from build123d import *

# Parameters (mm, degrees)
F1_DEPTH = 63.5
F0_W     = 25.4
F0_H     = 19.05
F2_DEPTH = 25.4
F3_DEPTH = 7.9375
F5_R     = 5.08
F6_DEPTH = 46.736


with BuildPart() as f1:
    # F0 (on Front) → F1 (new body, symmetric)
    with BuildSketch(Plane.XZ):
        Polygon((22.225, 9.525), (-41.275, 9.525), (-41.275, -9.525), (41.275, -9.525), (41.275, 9.525), align=None)
    extrude(amount=F1_DEPTH, both=True)

    # F0 (on Front) → F2 (join, symmetric)
    with BuildSketch(Plane.XZ):
        with BuildLine():
            Line((22.225, 27.0002), (22.225, 9.525))
            Line((22.225, 9.525), (41.275, 9.525))
            Line((41.275, 9.525), (41.275, 27.0002))
            ThreePointArc((41.275, 27.0002), (45.9246798487, 38.2255201513), (57.15, 42.8752))
            Line((57.15, 42.8752), (60.325, 42.8752))
            Line((60.325, 42.8752), (60.325, 61.9252))
            Line((60.325, 61.9252), (57.15, 61.9252))
            add(Edge.make_bspline(
                [(53.8854342407, 61.7722898912), (54.9842067368, 61.8365871986), (56.0728453275, 61.8876096574), (57.15, 61.9252)],
                knots=[108.5245810491, 108.5245810491, 108.5245810491, 108.5245810491, 111.5045361635, 111.5045361635, 111.5045361635, 111.5045361635], degree=3))
            ThreePointArc((53.8854342407, 61.7722898912), (31.3258777096, 50.5133948686), (22.225, 27.0002))
        make_face()
        with Locations((73.025, 52.4002)):
            Rectangle(F0_W, F0_H)
    extrude(amount=F2_DEPTH, both=True)

    # F0 (on Front) → F3 (join, symmetric)
    with BuildSketch(Plane.XZ):
        with BuildLine():
            add(Edge.make_bspline(
                [(-41.275, 9.525), (-39.5856284224, 39.4828766469), (13.870125209, 59.4306981306), (53.8854342407, 61.7722898912)],
                knots=[0, 0, 0, 0, 108.5245810491, 108.5245810491, 108.5245810491, 108.5245810491], degree=3))
            Line((-41.275, 9.525), (22.225, 9.525))
            Line((22.225, 9.525), (22.225, 27.0002))
            ThreePointArc((22.225, 27.0002), (31.3258777096, 50.5133948686), (53.8854342407, 61.7722898912))
        make_face()
    extrude(amount=F3_DEPTH, both=True)

    # F0 (on Front) → F4 (revolve)
    with BuildSketch(Plane.XZ):
        Polygon((85.725, 66.675), (85.725, 61.9252), (85.725, 42.8752), (85.725, 38.1), (111.125, 38.1), (111.125, 66.675), align=None)
    revolve(axis=Axis((85.725, 0, 52.3875), (0, 0, 1)))

    # F5
    f5_edges = [f1.edges().sort_by_distance(p)[0] for p in [
        (41.275, -63.5, 0),
        (-41.275, -63.5, 0),
        (41.275, 63.5, 0),
        (-41.275, 63.5, 0),
    ]]
    fillet(f5_edges, radius=F5_R)

    # F6 (add): a face of the model
    f6_faces = [f1.faces().sort_by_distance(p)[0] for p in [
        (85.725, 0, 38.1),
    ]]
    extrude(f6_faces, amount=F6_DEPTH)


solid = f1.part
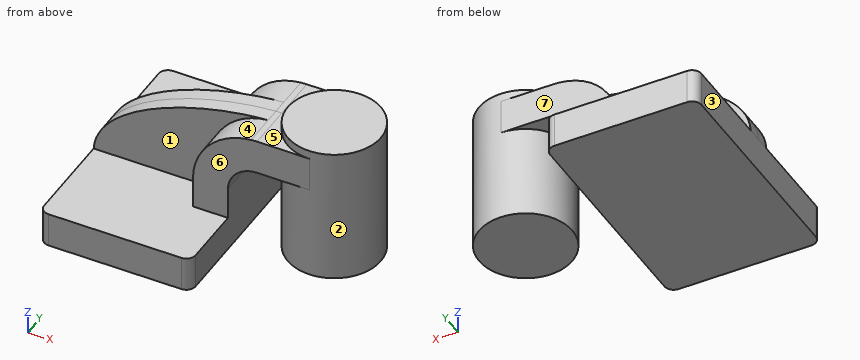
Check sheet for the modelled part. Datum: model origin and axes. Units: mm. Face numbers are marked on the shaded views. A direction names the side the tool comes from. Round coordinates to 2 decimals unless told otherwise and drop trailing zeros. Loops run counter-clockwise (first coordinate to the right, second up) from the corner with the lowest first, then second, coordinate; pieces in that order, holes last.
1. Set-up check for the marked faces 4, 5, 6 and 7: record each of +Z, -Z, +X, -X, +Y, -Y from which the full face is reachable in a straight line by a thin tool's end or side.
2. Mould release check, pull along X, two halves, no side actions. Record for the marked faces 1, 2 and 3: released by +X, released by -X, zero draft, split by the parting line, or undercut.
3. Scan lines: probe 1 along X at (y, z) = (26, -2) (3 decimals); probe 2 along Z at (x, y) = (29.5, -43) (3 decimals); probe 3 along Y at (x, z) = (81, 47.5). Record each from-to range of solid material in increasing order.
4. Sectioned sample at A-A on z = -3.5. Record the boundary of the cut face in (x, y) (3 decimals).
5. Gauge pin test, flat ends, axial feed: pin 1 Ø15.5 at (x, z) = (-8, 23.5) entering from -Y; pin 2 Ø6 at (x, z) = (72, 49) entering from +Y; pin 3 Ø4 at (x, y) = (29, 23) entering from +Z. Record the tip position at first contact, or that the pin passes through.
6. Sectioned sample at B-B on x = 71. Record the boundary of the cut face in (y, z) (3 decimals).
7. Sectioned sample at C-C on y = -33.5. Record the boundary of the cut face in (x, z) (3 decimals).
Recorded:
1. face 4: +Z, -X, -Y
1. face 5: +Z, -X
1. face 6: +Z, +X, -X, -Y
1. face 7: +Z, +X, -X, +Y
2. face 1: zero draft
2. face 2: undercut
2. face 3: released by -X
3. probe 1: x = -41.275 to 41.275
3. probe 2: z = -9.525 to 9.525
3. probe 3: y = -25.4 to 25.4
4. outline: (-41.275, -58.42) arc R5.08 ccw to (-36.195, -63.5) - (36.195, -63.5) arc R5.08 ccw to (41.275, -58.42) - (41.275, 58.42) arc R5.08 ccw to (36.195, 63.5) - (-36.195, 63.5) arc R5.08 ccw to (-41.275, 58.42) - close; circle Ø50.8 at (85.725, 0)
5. pin 1: stops at y = -7.94
5. pin 2: stops at y = 25.4
5. pin 3: stops at z = 50.15
6. outline: (-25.4, 42.875) - (-20.696, 42.875) - (-20.696, -8.636) - (20.696, -8.636) - (20.696, 42.875) - (25.4, 42.875) - (25.4, 61.925) - (20.696, 61.925) - (20.696, 66.675) - (-20.696, 66.675) - (-20.696, 61.925) - (-25.4, 61.925) - close
7. outline: (-41.275, -9.525) - (41.275, -9.525) - (41.275, 9.525) - (-41.275, 9.525) - close
